```python
from build123d import *

# Parameters (mm, degrees)
SKETCH1_R                       = 22.5
BOSS_EXTRUDE1_DEPTH             = 18
SKETCH2_W                       = 2
SKETCH2_H                       = 1.5
SKETCH2_W_2                     = 5
SKETCH2_H_2                     = 0.1
SKETCH3_R                       = 19.8375
BOSS_EXTRUDE2_DEPTH             = 3
SKETCH4_R                       = 3
BOSS_EXTRUDE3_DEPTH             = 15
BOSS_EXTRUDE4_START             = 10
SKETCH5_R                       = 3
BOSS_EXTRUDE4_DEPTH             = 10
CHAMFER1_SIZE                   = 0.5
M3X0_5_TAPPED_HOLE1_D           = 2.5
M3X0_5_TAPPED_HOLE1_DEPTH       = 4
BOSS_EXTRUDE5_DEPTH             = 23.5
SKETCH11_R                      = 0.7
BOSS_EXTRUDE6_DEPTH             = 2
SKETCH12_R                      = 0.9
BOSS_EXTRUDE7_DEPTH             = 1
CIRPATTERN1_COUNT               = 2
CIRPATTERN1_ANGLE               = 20
CIRPATTERN1_THE_OTHER_WAY_COUNT = 2
CIRPATTERN1_THE_OTHER_WAY_ANGLE = 20


with BuildPart() as part:
    # Sketch1 → Boss-Extrude1 (new body)
    with BuildSketch(Plane.XY):
        Circle(SKETCH1_R)
    extrude(amount=BOSS_EXTRUDE1_DEPTH)

    # Sketch2 → Cut-Revolve1 (revolve, cut)
    with BuildSketch(Plane(origin=(0, 0, 0), x_dir=(0, 0, -1), z_dir=(1, 0, 0)), mode=Mode.PRIVATE) as cut_revolve1_sk:
        with Locations((-15, 21.75)):
            Rectangle(SKETCH2_W, SKETCH2_H)
        with Locations((-10.5, 22.45)):
            Rectangle(SKETCH2_W_2, SKETCH2_H_2)
    revolve(cut_revolve1_sk.sketch.rotate(Axis((0, 0, 18), (0, 0, -1)), 180), axis=Axis((0, 0, 18), (0, 0, -1)), mode=Mode.SUBTRACT)

    # Sketch3 → Boss-Extrude2 (add)
    with BuildSketch(Plane.XY.offset(18)):
        Circle(SKETCH3_R)
    extrude(amount=BOSS_EXTRUDE2_DEPTH)

    # Sketch4 → Boss-Extrude3 (add)
    with BuildSketch(Plane.XY.offset(21)):
        Circle(SKETCH4_R)
    extrude(amount=BOSS_EXTRUDE3_DEPTH)

    # Sketch5 → Boss-Extrude4 (add)
    with BuildSketch(Plane(origin=(0, 0, 0), x_dir=(-1, 0, 0), z_dir=(0, 0, -1)).offset(BOSS_EXTRUDE4_START)):
        with Locations(Location((0, 0, 0), (0, 0, 180))):
            Circle(SKETCH5_R)
    extrude(amount=-BOSS_EXTRUDE4_DEPTH)

    # Chamfer1
    chamfer1_edges = [part.edges().sort_by_distance(p)[0] for p in [
        (-3, 0, 36),
        (-3, 0, -10),
    ]]
    chamfer(chamfer1_edges, length=CHAMFER1_SIZE)

    # M3x0.5 Tapped Hole1
    with Locations(Plane.XY.offset(21)):
        with Locations((12.990381057, 7.5), (0, -15), (-12.990381057, 7.5)):
            Hole(M3X0_5_TAPPED_HOLE1_D / 2, depth=M3X0_5_TAPPED_HOLE1_DEPTH)

    # Sketch10 → Boss-Extrude5 (add)
    with BuildSketch(Plane(origin=(0, 0, 0), x_dir=(1, 0, 0), z_dir=(0, 1, 0))):
        Polygon((1.154700538, -10.5), (0.577350269, -9.5), (-0.577350269, -9.5), (-1.154700538, -10.5), (-0.577350269, -11.5), (0.577350269, -11.5), align=None)
    boss_extrude5 = extrude(amount=BOSS_EXTRUDE5_DEPTH)

    # Sketch11 → Boss-Extrude6 (add)
    with BuildSketch(Plane(origin=(0, 23.5, 0), x_dir=(1, 0, 0), z_dir=(0, 1, 0))):
        with Locations(Location((0, -10.5, 0), (0, 0, 270))):
            Circle(SKETCH11_R)
    boss_extrude6 = extrude(amount=BOSS_EXTRUDE6_DEPTH)

    # Sketch12 → Boss-Extrude7 (add)
    with BuildSketch(Plane(origin=(0, 25.5, 0), x_dir=(1, 0, 0), z_dir=(0, 1, 0))):
        with Locations(Location((0, -10.5, 0), (0, 0, 270))):
            Circle(SKETCH12_R)
    boss_extrude7 = extrude(amount=BOSS_EXTRUDE7_DEPTH)

    # CirPattern1: Boss-Extrude5, Boss-Extrude6, Boss-Extrude7 ×2 about axis
    cirpattern1_axis = Axis((0, 0, 0), (0, 0, 1))
    add([boss_extrude5.rotate(cirpattern1_axis, i * CIRPATTERN1_ANGLE / (CIRPATTERN1_COUNT - 1)) for i in range(1, CIRPATTERN1_COUNT)])
    add([boss_extrude6.rotate(cirpattern1_axis, i * CIRPATTERN1_ANGLE / (CIRPATTERN1_COUNT - 1)) for i in range(1, CIRPATTERN1_COUNT)])
    add([boss_extrude7.rotate(cirpattern1_axis, i * CIRPATTERN1_ANGLE / (CIRPATTERN1_COUNT - 1)) for i in range(1, CIRPATTERN1_COUNT)])

    # CirPattern1 the other way: Boss-Extrude5, Boss-Extrude6, Boss-Extrude7 ×2 about axis
    cirpattern1_the_other_way_axis = Axis((0, 0, 0), (0, 0, -1))
    add([boss_extrude5.rotate(cirpattern1_the_other_way_axis, i * CIRPATTERN1_THE_OTHER_WAY_ANGLE / (CIRPATTERN1_THE_OTHER_WAY_COUNT - 1)) for i in range(1, CIRPATTERN1_THE_OTHER_WAY_COUNT)])
    add([boss_extrude6.rotate(cirpattern1_the_other_way_axis, i * CIRPATTERN1_THE_OTHER_WAY_ANGLE / (CIRPATTERN1_THE_OTHER_WAY_COUNT - 1)) for i in range(1, CIRPATTERN1_THE_OTHER_WAY_COUNT)])
    add([boss_extrude7.rotate(cirpattern1_the_other_way_axis, i * CIRPATTERN1_THE_OTHER_WAY_ANGLE / (CIRPATTERN1_THE_OTHER_WAY_COUNT - 1)) for i in range(1, CIRPATTERN1_THE_OTHER_WAY_COUNT)])


solid = part.part
```
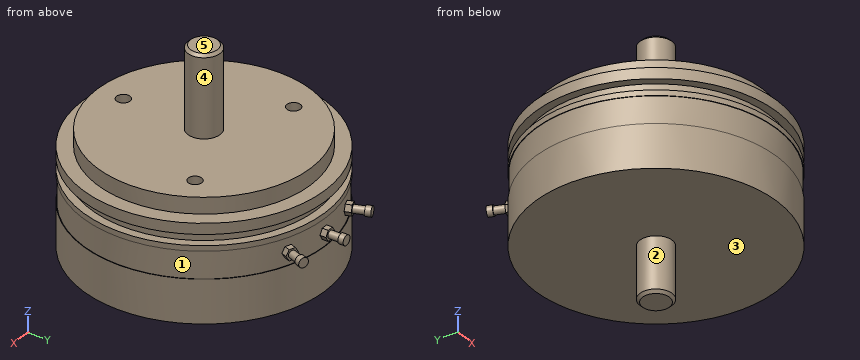
For this review, take the finished solid that the model builds, in its own axes (mm). Face numbers are marked on the shaded views. A direction names the side the tool comes from. Coordinates: 2 decimals unless noted, no trailing zeros. Order: outer loops, then holes, each group sorted by start corner. A loop starts at its lowest first (then second) coordinate and runs counter-clockwise, first axis right, second up. Notation, with made-up numbers: (0, 61) -> (36, 61) arc R24 cw to (36, 84) -> close; hole circle Ø3 at (-2.75, -5.75). An arc over 180 degrees is marked (long way). Use CSV: the item, a comma, the result in double quotes. Start each with the question number.
Item 1: Wall thickness on probe 1 along Y at (x, z) = (0, 19.65); probe 2 along Z at (x, y) = (13, -12); probe 3 along Z at (x, y) = (-16.5, 14): over which ranges is each line inside the solid? List them lowest first.
Item 2: Draft analysis for pull direction Z (two halves, no side actions). For the marked faces 1, 2 and 3, state which applies: pulls with the +Z half, pulls with the -Z half, needs draft (parallel to the pull), parting line crosses it, or undercut.
Item 3: We need section D-D, the plane z = 20. Give the number of separate pieces and of enclosed holes in the cut face, then the cut area to 3 significant figures.
Item 4: Insertion check: pin 1 (1 mm diameter, centred on x = -12.5, y = -5, fed in from +Z); pin 2 (0.8 mm diameter, centred on x = 13, y = 8, fed in from +Z); pin 3 (0.9 mm diameter, centred on x = 0, y = 23, fed in from +Z). Each pin has a flat end and moves straight along its axis. Give the tip position at first contact, or say it passes through.
Item 5: We need section C-C, the plane x = -13. Give the boundary of the cut face in (y, z), then the cut area to 3 significant figures.
Item 6: For the marked faces 4 and 5, list the 3-axis set-ups (+Z, -Z, +X, -X, +Y, -Y) from which the entire face can be reached by the end or side of a thin tool; tool diameter is ignored.
Item 7: We need section B-B, the plane z = 4. Give the boundary of the cut face in (x, y).
Item 8: We need section A-A, the plane y = 5.5. Give the boundary of the cut face in (x, z), then the cut area to 3 significant figures.
Derived:
1,probe 1,"y = -19.84 to -16.25, -13.75 to 19.84"
1,probe 2,"z = 0 to 21"
1,probe 3,"z = 0 to 14, 16 to 18"
2,face 1,"undercut"
2,face 2,"needs draft"
2,face 3,"pulls with the -Z half"
3,separate pieces,"1"
3,enclosed holes,"3"
3,area,"1,220 mm^2"
4,pin 1,"stops at z = 21"
4,pin 2,"stops at z = 17"
4,pin 3,"stops at z = 11.5"
5,outline,"(-18.36, 0) -> (18.36, 0) -> (18.36, 8) -> (18.24, 8) -> (18.24, 13) -> (18.36, 13) -> (18.36, 14) -> (16.49, 14) -> (16.49, 16) -> (18.36, 16) -> (18.36, 18) -> (14.98, 18) -> (14.98, 21) -> (8.75, 21) -> (8.75, 17) -> (6.25, 17) -> (6.25, 21) -> (-14.98, 21) -> (-14.98, 18) -> (-18.36, 18) -> (-18.36, 16) -> (-16.49, 16) -> (-16.49, 14) -> (-18.36, 14) -> (-18.36, 13) -> (-18.24, 13) -> (-18.24, 8) -> (-18.36, 8) -> close"
5,area,"732 mm^2"
6,face 4,"+Z"
6,face 5,"+Z, +X, -X, +Y, -Y"
7,outline,"circle Ø45 at (0, 0)"
8,outline,"(-21.82, 0) -> (21.82, 0) -> (21.82, 8) -> (21.71, 8) -> (21.71, 13) -> (21.82, 13) -> (21.82, 14) -> (20.27, 14) -> (20.27, 16) -> (21.82, 16) -> (21.82, 18) -> (19.06, 18) -> (19.06, 21) -> (-19.06, 21) -> (-19.06, 18) -> (-21.82, 18) -> (-21.82, 16) -> (-20.27, 16) -> (-20.27, 14) -> (-21.82, 14) -> (-21.82, 13) -> (-21.71, 13) -> (-21.71, 8) -> (-21.82, 8) -> close"
8,area,"893 mm^2"
